Verification items for the finished model (mm, model axes). Face numbers are marked on the shaded views. A direction names the side the tool comes from. Round coordinates to 2 decimals unless told otherwise and drop trailing zeros. Order: outer loops, then holes, each group sorted by start corner. A loop starts at its lowest first (then second) coordinate and runs counter-clockwise, first axis right, second up. Notation, with made-up numbers: M 87,44.25 L 117,44.25 A30 ccw 117,79.25 Z; hole C -17,27.25 d11. An arc over 180 degrees is marked long. Use one line per item in the form item = value. Start each with the question number.
Item 1: Cross-section at D-D on y = 0. Count the separate pieces of the cut face and the enclosed holes in it, then the cut area to 3 significant figures.
Item 2: Thickness scan on probe 1 along Y at (x, z) = (80, 5.5); probe 2 along X at (y, z) = (-0.75, 7.25); probe 3 along Y at (x, z) = (-29, 4.25). Record the ranges inside material, lowest first. Write a range as [from, to].
Item 3: Go/stop test with flat-tipped pins: pin 1 Ø1 at (x, z) = (-9.5, 1) entering from +Y; pin 2 Ø7.5 at (x, y) = (-80, 0) entering from +Z; pin 3 Ø4.5 at (x, y) = (80, 0) entering from -Z; pin 4 Ø1.5 at (y, z) = (10, 9) entering from +X. Record where each tip stops, or that it passes through.
Item 4: Tool access check on the marked faces 5 and 6. Record the directions out of +Z, -Z, +X, -X, +Y, -Y that give a thin tool (end or side, any length) a straight path to the whole face; none if there is none.
Item 5: Release check for a two-part mould opening along X. For the marked faces 1, 2, 3 and 4 record: +X half, -X half, draft (parallel to the pull), parting line (faces both ways), or undercut.
Item 6: Cross-section at A-A on x = -80. Enter the section's corners in (y, z).
Item 7: Cross-section at C-C on x = 29. Enter the section's corners in (y, z), then the cut area to 3 significant figures.
Item 8: Cross-section at B-B on z = 7.5. Enter the section's corners in (x, y).
Autodesk Inventor part; units mm, degrees
ref_plane "YZ Plane" through (0, 0, 0) normal (1, 0, 0) x (0, 1, 0)
ref_plane "XZ Plane" through (0, 0, 0) normal (0, 1, 0) x (-1, 0, 0)
ref_plane "XY Plane" through (0, 0, 0) normal (0, 0, 1) x (1, 0, 0)
sketch "Sketch1" plane through (0, 0, 0) normal (0, 0, 1) x (1, 0, 0)
  line L0 (-90, -12.5) -> (90, -12.5)
  line L1 (90, -12.5) -> (90, 12.5)
  line L2 (90, 12.5) -> (-90, 12.5)
  line L3 (-90, 12.5) -> (-90, -12.5)
  line L4 (-90, -12.5) -> (90, 12.5) construction
  line L5 (90, -12.5) -> (-90, 12.5) construction
  line L6 (-246.96, 0) -> (246.96, 0) construction
  circle A0 centre (-80, 0) radius 2.9
  line L7 (0, 17.5) -> (0, -17.5) construction
  line L8 (246.96, 0) -> (-246.96, 0) construction
  circle A1 centre (80, 0) radius 2.9
  point P0 (0, 0)
  dimension "d0" = 25
  dimension "d1" = 180
  dimension "d2" = 5.8
  dimension "d3" = 160
extrude "Extrusion1" add sketch "Sketch1" along normal blind 10
sketch "Sketch2" plane through (0, 0, 10) normal (0, 0, 1) x (1, 0, 0)
  line L0 (90, 12.5) -> (-90, 12.5)
  line L1 (-65, 12.5) -> (65, 12.5)
  line L2 (65, 12.5) -> (65, -2.5)
  line L3 (65, -2.5) -> (-65, -2.5)
  line L4 (-65, -2.5) -> (-65, 12.5)
  line L5 (-90, 12.5) -> (-90, -12.5)
  line L6 (90, -12.5) -> (90, 12.5)
  line L7 (-90, -12.5) -> (90, -12.5)
  point P0 (0, 0)
  dimension "d6" = 25
  dimension "d7" = 25
  dimension "d8" = 10
extrude "Extrusion2" cut sketch "Sketch2" against normal through all contours L2 L3 L4 L0
fillet "Fillet1" radius 5 8 edges at (-65, -2.5, 5) (-65, 12.5, 5) (-90, 12.5, 5) (-90, -12.5, 5) (90, -12.5, 5) (90, 12.5, 5) (65, 12.5, 5) (65, -2.5, 5)
chamfer "Chamfer1" distance 0.8 angle 45 32 edges at (0, -2.5, 0) (63.5355, -1.0355, 0) (65, 5, 0) (66.4645, 11.0355, 0) (77.5, 12.5, 0) (88.5355, 11.0355, 0) (90, 0, 0) (88.5355, -11.0355, 0) (0, -12.5, 0) (-88.5355, -11.0355, 0) (-90, 0, 0) (-88.5355, 11.0355, 0) (-77.5, 12.5, 0) (-66.4645, 11.0355, 0) (-65, 5, 0) (-63.5355, -1.0355, 0) (0, -2.5, 10) (-63.5355, -1.0355, 10) (-65, 5, 10) (-66.4645, 11.0355, 10) (-77.5, 12.5, 10) (-88.5355, 11.0355, 10) (-90, 0, 10) (-88.5355, -11.0355, 10) (0, -12.5, 10) (88.5355, -11.0355, 10) (90, 0, 10) (88.5355, 11.0355, 10) (77.5, 12.5, 10) (66.4645, 11.0355, 10) (65, 5, 10) (63.5355, -1.0355, 10)
properties part number "DisplayHolder_3DPrint"
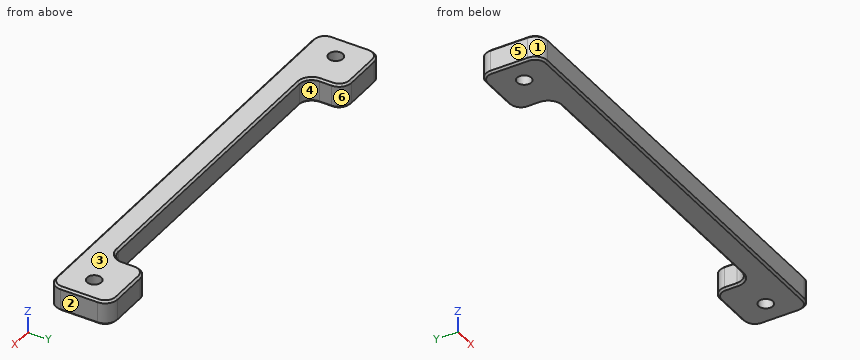
Output values:
q1.separate_pieces = 4
q1.enclosed_holes = 0
q1.area = 395 mm2
q2.probe_1 = [-12.5, -2.9], [2.9, 12.5]
q2.probe_2 = [-90, -82.8], [-77.2, -63.8], [63.8, 77.2], [82.8, 90]
q2.probe_3 = [-12.5, -2.5]
q3.pin_1 = -2.5
q3.pin_2 = 10
q3.pin_3 = through
q3.pin_4 = 89.68
q4.face_5 = +Z, -Z, -X, +Y, -Y
q4.face_6 = +Z, -Z, +Y
q5.face_1 = -X half
q5.face_2 = +X half
q5.face_3 = draft
q5.face_4 = undercut
q6.outline = M -12.5,0.8 L -11.7,0 L -2.9,0 L -2.9,10 L -11.7,10 L -12.5,9.2 Z; M 2.9,0 L 11.7,0 L 12.5,0.8 L 12.5,9.2 L 11.7,10 L 2.9,10 Z
q7.outline = M -12.5,0.8 L -11.7,0 L -3.3,0 L -2.5,0.8 L -2.5,9.2 L -3.3,10 L -11.7,10 L -12.5,9.2 Z
q7.area = 98.7 mm2
q8.outline = M -90,-7.5 A5 ccw -85,-12.5 L 85,-12.5 A5 ccw 90,-7.5 L 90,7.5 A5 ccw 85,12.5 L 70,12.5 A5 ccw 65,7.5 L 65,2.5 A5 cw 60,-2.5 L -60,-2.5 A5 cw -65,2.5 L -65,7.5 A5 ccw -70,12.5 L -85,12.5 A5 ccw -90,7.5 Z; hole C -80,0 d5.8; hole C 80,0 d5.8
